Source: CAD feature listing. Evaluate the final solid. Frame: model axes, mm. Coordinates: 2 decimals unless noted, no trailing zeros. Order: outer loops, then holes, each group sorted by start corner. A loop starts at its lowest first (then second) coordinate and runs counter-clockwise, first axis right, second up. Notation, with made-up numbers: (-3, 53.25) -> (56, 53.25) arc R29 cw to (56, 92.25) -> close; hole circle Ø4 at (35.5, 59). An arc over 180 degrees is marked (long way). Write item = value, one per line. Start each with the question number.
Item 1: Section query D-D (z = 70). Output: boundary loops of the cut face in (x, y), then the cut area to 3 significant figures.
Item 2: Section query C-C (y = 1.65). Output: boundary loops of the cut face in (x, z), then the cut area to 3 significant figures.
Item 3: Section query B-B (x = -7.5). Output: boundary loops of the cut face in (y, z).
Item 4: Section query A-A (z = 31). Output: boundary loops of the cut face in (x, y), then the cut area to 3 significant figures.
Item 5: Ray query, line 1 along X through (y, z) = (1.95, 24); line 2 along Z through (x, y) = (37.5, 1.4); line 3 along Z through (x, y) = (50, 1.6). Return the intervals inside material, ascending. Write a range as [from, to].
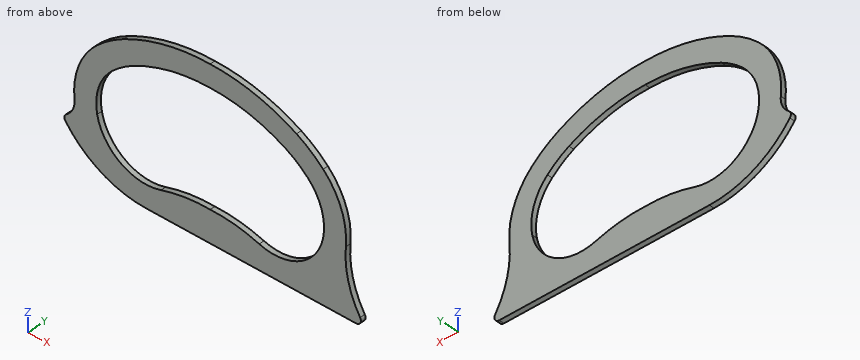
```python
from build123d import *

# Parameters (mm, degrees)
BOSS_EXTRUDE1_DEPTH = 3


with BuildPart() as part:
    # Sketch1 → Boss-Extrude1 (new body)
    with BuildSketch(Plane(origin=(0, 0, 0), x_dir=(1, 0, 0), z_dir=(0, 1, 0))):
        with BuildLine():
            Line((-31.744728966, 17.146847669), (90.112594835, 17.146847669))
            ThreePointArc((90.112594835, 17.146847669), (92.565620931, 15.696908028), (92.478118614, 12.848749793))
            ThreePointArc((92.478118614, 12.848749793), (85.55789243, -3.426446533), (84.197045341, -21.059360105))
            ThreePointArc((84.197045341, -21.059360105), (81.584356476, -40.056839396), (71.059546267, -56.086771791))
            ThreePointArc((71.059546267, -56.086771791), (63.736401413, -62.212035121), (55.619101507, -67.237643905))
            ThreePointArc((55.619101507, -67.237643905), (31.315398674, -76.373966348), (5.514443068, -79.281379121))
            ThreePointArc((5.514443068, -79.281379121), (-20.286512537, -76.373966348), (-44.59021537, -67.237643905))
            ThreePointArc((-44.59021537, -67.237643905), (-52.707515276, -62.212035121), (-60.03066013, -56.086771791))
            ThreePointArc((-60.03066013, -56.086771791), (-70.666595812, -39.757213537), (-73.108914698, -20.422977605))
            ThreePointArc((-73.108914698, -20.422977605), (-74.05774513, -14.573171652), (-77.796738294, -9.975298341))
            ThreePointArc((-77.796738294, -9.975298341), (-78.92336426, -8.119267018), (-78.384627262, -6.015959912))
            ThreePointArc((-78.384627262, -6.015959912), (-57.78218164, 11.037323217), (-31.744728966, 17.146847669))
        make_face()
        with BuildLine():
            ThreePointArc((5.514443068, -1.081998552), (19.929462064, -0.256796987), (34.001578397, 2.975736417))
            ThreePointArc((34.001578397, 2.975736417), (57.41708067, 0.337527336), (70.993213533, -18.922132846))
            ThreePointArc((70.993213533, -18.922132846), (70.131692962, -34.019755233), (62.170548913, -46.876683515))
            ThreePointArc((62.170548913, -46.876683515), (56.242369759, -51.835162299), (49.671311961, -55.903456704))
            ThreePointArc((49.671311961, -55.903456704), (28.252463685, -63.945588922), (5.514443068, -66.480420375))
            ThreePointArc((5.514443068, -66.480420375), (-17.223577548, -63.945588922), (-38.642425824, -55.903456704))
            ThreePointArc((-38.642425824, -55.903456704), (-45.213483622, -51.835162299), (-51.141662776, -46.876683515))
            ThreePointArc((-51.141662776, -46.876683515), (-59.102806825, -34.019755233), (-59.964327396, -18.922132846))
            ThreePointArc((-59.964327396, -18.922132846), (-46.388194533, 0.337527336), (-22.97269226, 2.975736417))
            ThreePointArc((-22.97269226, 2.975736417), (-8.900575928, -0.256796987), (5.514443068, -1.081998552))
        make_face(mode=Mode.SUBTRACT)
    extrude(amount=BOSS_EXTRUDE1_DEPTH)


solid = part.part
```
Computed:
q1.outline = (-38.92, 0) -> (49.95, 0) -> (49.95, 3) -> (-38.92, 3) -> close
q1.area = 267 mm^2
q2.outline = (-78.38, 6.02) arc R58.54 ccw to (-31.74, -17.15) -> (90.11, -17.15) arc R2.8 ccw to (92.48, -12.85) arc R54.65 cw to (84.2, 21.06) arc R43.52 ccw to (71.06, 56.09) arc R67.2 ccw to (55.62, 67.24) arc R105.23 ccw to (5.51, 79.28) arc R105.23 ccw to (-44.59, 67.24) arc R67.2 ccw to (-60.03, 56.09) arc R43.52 ccw to (-73.11, 20.42) arc R11.48 cw to (-77.8, 9.98) arc R2.8 ccw to start; hole (-59.96, 18.92) arc R28.75 ccw to (-22.97, -2.98) arc R85.73 cw to (5.51, 1.08) arc R85.73 cw to (34, -2.98) arc R28.75 ccw to (70.99, 18.92) arc R30.72 ccw to (62.17, 46.88) arc R54.4 ccw to (49.67, 55.9) arc R92.43 ccw to (5.51, 66.48) arc R92.43 ccw to (-38.64, 55.9) arc R54.4 ccw to (-51.14, 46.88) arc R30.72 ccw to start
q2.area = 5,750 mm^2
q3.outline = (0, -17.15) -> (3, -17.15) -> (3, 0.44) -> (0, 0.44) -> close; (0, 65.73) -> (3, 65.73) -> (3, 78.62) -> (0, 78.62) -> close
q4.outline = (-72.88, 0) -> (-59.89, 0) -> (-59.89, 3) -> (-72.88, 3) -> close; (70.92, 0) -> (83.91, 0) -> (83.91, 3) -> (70.92, 3) -> close
q4.area = 77.9 mm^2
q5.line_1 = [-73.32, -60.52], [71.55, 84.35]
q5.line_2 = [-17.15, -3.86], [61.21, 74.69]
q5.line_3 = [-17.15, -3.42], [55.73, 69.98]
